Here's how the part is built. I have some questions about the finished solid (model axes, mm). A direction names the side the tool comes from. Give positions to 0.01 mm unless a question says otherwise; leave off trailing zeros. Write each loop counter-clockwise with the first axis right and the second up, starting at its lowest first coordinate (ties: lowest second). Pieces come first, ordered by that corner, then holes. Notation, with made-up numbers: (65, 5) -> (111, 5) arc R26 ccw to (111, 34) -> close; hole circle Ø10 at (4.25, -38). An arc over 180 degrees is marked (long way). Use CSV: the item, a comma, the result in double quotes. Start each with the question number.
(1) I need wall thicknesses on L1, parallel to Y at x = 97, z = -8.75; L2, parallel to Y at x = 102, z = -3; L3, parallel to Y at x = 84, z = -1. Which ranges of each line are inside material? Lowest first, please. Write a range as [from, to].
(2) If we mould it in two halves opening along Y, with no side actions, what happens to faces 4 (the cylindrical face through (116.54, 63.28, -7.4)), 5 (the cylindrical face through (83.656, -12.347, -7.395)), 6 (the cylindrical face through (97.57, 52.28, -7.4)), 7 (the flat face through (111, 13, 0))? For each: pulls with the +Y half, pulls with the -Y half, needs draft (parallel to the pull), parting line crosses it, or undercut.
(3) Which directions (+Z, -Z, +X, -X, +Y, -Y) give clear straight access to the entire face, cutting with the end or side of a thin tool? Please do faces 1 (the flat face through (89.476, -11.088, -7.395)), 2 (the flat face through (85.89, 13.75, -7.4)), 3 (the flat face through (78.34, -0.74, -7.4)).
(4) Suppose I cut it at A-A on z = -4.25. List the corners of the cut face in (x, y) for me.
(5) Suppose I cut it at C-C on y = -6.5. List the corners of the cut face in (x, z) for me.
(6) Suppose I cut it at B-B on x = 83.5. List the corners of the cut face in (y, z) for me, plus the area to 3 significant figures.
(7) For pin 1 Ø3 at (x, z) = (125.5, -6) entering from -Y; pin 2 Ø5 at (x, z) = (89, -2) entering from +Y; pin 3 Ø8 at (x, z) = (103.5, -3) entering from +Y, each with a flat end and sliding along its axis, tell me the tip position at first contact or that it passes through.
from build123d import *

# Parameters (mm, degrees)
DODANIE_WYCI_GNI_CIE1_DEPTH = 15


with BuildPart() as part:
    # Szkic2 → Dodanie-wyciągnięcie1 (new body)
    with BuildSketch(Plane(origin=(0, 0, 0), x_dir=(-1, 0, 0), z_dir=(0, 0, -1))):
        with BuildLine():
            Line((-74.826032056, 11.014530402), (-81.951422725, -12.818572719))
            ThreePointArc((-81.951422725, -12.818572719), (-83.679858685, -12.341119841), (-85.426816489, -11.936656557))
            Line((-85.426816489, -11.936656557), (-93.639920436, -10.215979742))
            ThreePointArc((-93.639920436, -10.215979742), (-105.622705702, -13.873790687), (-108.951787413, -25.952033051))
            ThreePointArc((-108.951787413, -25.952033051), (-107.042286981, -32.953737236), (-104.683334782, -39.817074466))
            Line((-104.683334782, -39.817074466), (-125.246132685, -47.638285521))
            ThreePointArc((-125.246132685, -47.638285521), (-133.907193125, 4.986344284), (-121.356345693, 56.821099602))
            ThreePointArc((-121.356345693, 56.821099602), (-116.45353268, 63.356793916), (-109.346193532, 67.386509274))
            ThreePointArc((-109.346193532, 67.386509274), (-102.153493063, 69.460884834), (-94.851646537, 71.110433658))
            Line((-94.851646537, 71.110433658), (-91.74794023, 55.218917354))
            ThreePointArc((-91.74794023, 55.218917354), (-97.643827413, 52.217038431), (-101.674756414, 46.970670723))
            ThreePointArc((-101.674756414, 46.970670723), (-104.340687454, 40.706522101), (-106.621107385, 34.291973698))
            ThreePointArc((-106.621107385, 34.291973698), (-105.521825108, 23.188783802), (-96.655711946, 16.415211274))
            Line((-96.655711946, 16.415211274), (-74.826032056, 11.014530402))
        make_face()
    extrude(amount=DODANIE_WYCI_GNI_CIE1_DEPTH)


solid = part.part
Geometry says:
1,L1,"[-9.96, 16.51], [52.72, 70.67]"
1,L2,"[-11.25, 19.04], [46.26, 69.5]"
1,L3,"[-12.26, 13.28]"
2,face 4,"pulls with the +Y half"
2,face 5,"pulls with the -Y half"
2,face 6,"undercut"
2,face 7,"needs draft"
3,face 1,"+Z, -Z, -Y"
3,face 2,"+Z, -Z, -X"
3,face 3,"+Z, -Z, -X, -Y"
4,outline,"(74.83, 11.01) -> (81.95, -12.82) arc R42.7 cw to (85.43, -11.94) -> (93.64, -10.22) arc R13 cw to (108.95, -25.95) arc R112 cw to (104.68, -39.82) -> (125.25, -47.64) arc R134 ccw to (121.36, 56.82) arc R20 ccw to (109.35, 67.39) arc R127.76 ccw to (94.85, 71.11) -> (91.75, 55.22) arc R15 cw to (101.67, 46.97) arc R112 cw to (106.62, 34.29) arc R14 cw to (96.66, 16.42) -> close"
5,outline,"(80.06, -15) -> (133.84, -15) -> (133.84, 0) -> (80.06, 0) -> close"
6,outline,"(-12.39, -15) -> (13.16, -15) -> (13.16, 0) -> (-12.39, 0) -> close"
6,area,"383 mm²"
7,pin 1,"y = -47.64"
7,pin 2,"y = 15.14"
7,pin 3,"y = 70.11"
